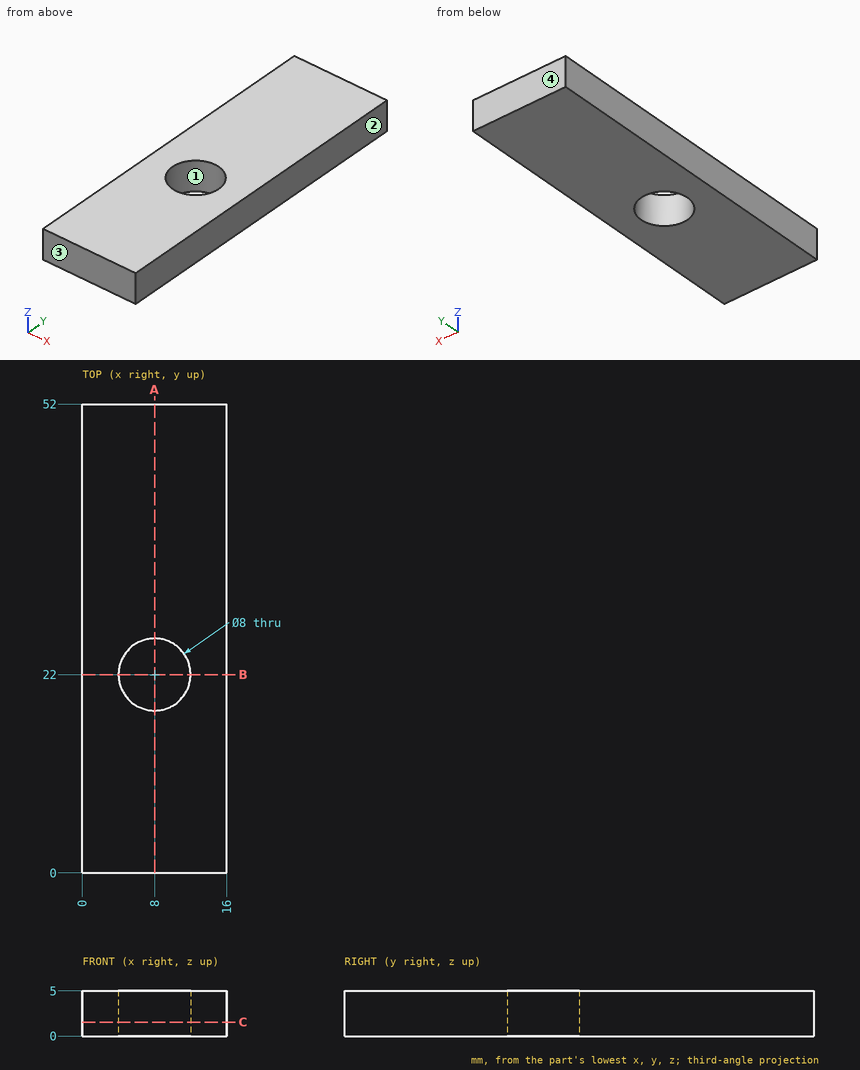
Geometry check sheet. Reference: drawing and pictorial views, mm from the part's lowest x, y, z. Coordinates: 2 decimals unless noted, no trailing zeros. Write each loop counter-clockwise with the first axis right and the second up, starting at its lowest first coordinate (ties: lowest second). Pieces come first, ordered by that corner, then holes. Notation, with made-up numbers: M 6.5,-37 L 42.5,-37 A10 ccw 42.5,-19 Z; hole C 75.5,-34 d5. An arc over 180 degrees is marked long. Write item = value, one per line. Start each with the question number.
1. Sectioned sample at B-B (y = 22). Record the cut outline in (x, z).
2. Thickness scan on probe 1 along Y at (x, z) = (8, 3.3); probe 2 along X at (y, z) = (19.5, 2.45); probe 3 along Y at (x, z) = (9.75, 4.75). Record the ranges inside material, lowest first.
3. Mould release check, pull along Y, two halves, no side actions. Record for the marked faces 1, 2, 3 and 4: pulls with the +Y half, pulls with the -Y half, needs draft (parallel to the pull), parting line crosses it, or undercut.
4. Sectioned sample at C-C (z = 1.55). Record the cut outline in (x, y), then the cut area to 3 significant figures.
5. Go/stop test with a flat-tipped pin: pin 1 (6 mm diameter, centred on x = 1.5, y = 7, fed in from -Z). Record where the tip stops, or that it passes through.
6. Sectioned sample at A-A (x = 8). Record the cut outline in (y, z).
The answers:
q1.outline = M 0,0 L 4,0 L 4,5 L 0,5 Z; M 12,0 L 16,0 L 16,5 L 12,5 Z
q2.probe_1 = 0 to 18, 26 to 52
q2.probe_2 = 0 to 4.88, 11.12 to 16
q2.probe_3 = 0 to 18.4, 25.6 to 52
q3.face_1 = undercut
q3.face_2 = needs draft
q3.face_3 = pulls with the -Y half
q3.face_4 = pulls with the +Y half
q4.outline = M 0,0 L 16,0 L 16,52 L 0,52 Z; hole C 8,22 d8
q4.area = 782 mm²
q5.pin_1 = 0
q6.outline = M 0,0 L 18,0 L 18,5 L 0,5 Z; M 26,0 L 52,0 L 52,5 L 26,5 Z
